The model under review builds one solid part; all positions refer to its coordinate system, in mm. A direction names the side the tool comes from. Give positions to 0.01 mm unless a question says otherwise; leave off trailing zeros. Loops run counter-clockwise (first coordinate to the right, second up) from the corner with the lowest first, then second, coordinate; pieces in that order, holes last. Notation, with made-up numbers: M -37.5,19 L -9.5,19 A23 cw -9.5,33 Z; hole C -8.75,42 d11. An arc over 180 degrees is marked long. One line per item, written item: value. Start each with the question number.
Q1. Mouldability with a two-part tool opening along X and no side actions: class faces 1 (the face through (0, 10, 0)), 2 (the face through (-1.5, -0.07, 0.49)), 3 (the face through (-3, 0.1, -0.2)), 4 (the face through (-0.195, 18.513, 0.486)) as released by +X, released by -X, zero draft, split by the parting line, or undercut.
Q2. We need section D-D on y = 11.25. Write out the cut boundary in (x, z), plus the area to 3 significant figures.
Q3. We need section B-B on x = 0.25. Write out the cut boundary in (y, z).
Q4. To check wall thickness, follow line 1 along Y through (x, z) = (0, -0.1); line 2 along Y through (x, z) = (0, 1); line 3 along Y through (x, z) = (0.5, 0.2). State the ranges of each line that lie inside material, in increasing order. Write a range as from..to.
Q5. We need section C-C on x = 2.5. Write out the cut boundary in (y, z), plus the area to 3 significant figures.
Q6. For pin 1 (3 mm diameter, centred on x = 1.5, y = 12.5, fed in from -Z); pin 2 (2.5 mm diameter, centred on x = 0, y = 20, fed in from -Z), all flat-tipped, find the tip position at first contact; note any pin that passes through.
Q7. For faces 5 (the face through (1.3, -1.3, -0.5)), 6 (the face through (-0.65, 17.07, -0.25)), list the 3-axis set-ups (+Z, -Z, +X, -X, +Y, -Y) from which the entire face can be reached by the end or side of a thin tool; tool diameter is ignored.
Q8. We need section A-A on z = 0.7. Write out the cut boundary in (x, y).
Autodesk Inventor part; units mm, degrees
ref_plane "YZ Plane" through (0, 0, 0) normal (1, 0, 0) x (0, 1, 0)
ref_plane "XZ Plane" through (0, 0, 0) normal (0, 1, 0) x (-1, 0, 0)
ref_plane "XY Plane" through (0, 0, 0) normal (0, 0, 1) x (1, 0, 0)
sketch "Skizze1" plane through (0, 0, 0) normal (0, 0, 1) x (1, 0, 0)
  line L0 (0, 31) -> (0, -11) construction
  line L1 (-7, 0) -> (7, 0) construction
  circle A0 centre (0, 0) radius 1.5
  arc A1 (-5, 0) -> (5, 0) centre (0, 0) ccw
  circle A2 centre (0, 20) radius 1.5
  arc A3 (5, 20) -> (-5, 20) centre (0, 20) ccw
  line L2 (-5, 20) -> (-5, 0)
  line L3 (5, 20) -> (5, 0)
  circle A4 centre (0, 0) radius 3
  circle A5 centre (0, 20) radius 3
  dimension "d0" = 3
  dimension "d1" = 10
  dimension "d4" = 1.5
  dimension "d7" = 20
extrude "Extrusion1" add sketch "Skizze1" along normal blind 1.5 contours L2 A3 L3 A1 | A4 | A5
extrude "Extrusion2" add sketch "Skizze1" against normal blind 0.5 contours A4 | A5
properties part number "Mouth-Lever"
Solved:
1. face 1: zero draft
1. face 2: undercut
1. face 3: split by the parting line
1. face 4: undercut
2. outline: M -5,0 L 5,0 L 5,1.5 L -5,1.5 Z
2. area: 15.0 mm2
3. outline: M -4.99,0 L -2.99,0 L -2.99,-0.5 L -1.48,-0.5 L -1.48,1.5 L -4.99,1.5 Z; M 1.48,-0.5 L 2.99,-0.5 L 2.99,0 L 17.01,0 L 17.01,-0.5 L 18.52,-0.5 L 18.52,1.5 L 1.48,1.5 Z; M 21.48,-0.5 L 22.99,-0.5 L 22.99,0 L 24.99,0 L 24.99,1.5 L 21.48,1.5 Z
4. line 1: -3..-1.5, 1.5..3, 17..18.5, 21.5..23
4. line 2: -5..-1.5, 1.5..18.5, 21.5..25
4. line 3: -4.97..-1.41, 1.41..18.59, 21.41..24.97
5. outline: M -4.33,0 L -1.66,0 L -1.66,-0.5 L 1.66,-0.5 L 1.66,0 L 18.34,0 L 18.34,-0.5 L 21.66,-0.5 L 21.66,0 L 24.33,0 L 24.33,1.5 L -4.33,1.5 Z
5. area: 46.3 mm2
6. pin 1: z = 0
6. pin 2: through
7. face 5: -Z, +X, -X, +Y, -Y
7. face 6: -Z
8. outline: M -5,0 A5 ccw 5,0 L 5,20 A5 ccw -5,20 Z; hole C 0,0 d3; hole C 0,20 d3
